CAD build for the part. Positions are in the model's coordinates, mm. A direction names the side the tool comes from. Round coordinates to 2 decimals unless told otherwise and drop trailing zeros. Write each loop counter-clockwise with the first axis right and the second up, starting at its lowest first coordinate (ties: lowest second). Pieces come first, ordered by that corner, then holes. Notation, with made-up numbers: (12, 15.25) - (37, 15.25) arc R19 ccw to (37, 47.25) - close; hole circle Ø6 at (45.25, -29.75). An arc over 180 degrees is marked (long way). Use one line per item in the form item = value. Start each with the question number.
Item 1: Drill centre line: L1, parallel to Z at x = -90, y = 5.75. Where is it in solid material? Low to high.
Item 2: Band-saw the part on A-A, the plane x = -224.5. List the corners of the cut face in (y, z).
Item 3: Pull direction X, two halves, no side cores. Call faces 1 (the flat face through (-108.74, 3, 73)), 2 (the flat face through (-357, 3, -69.85)), 3 (the flat face through (-360.818, 3, 1)): +X half, -X half, draft (parallel to the pull), parting line (faces both ways), or undercut.
Item 4: Pin check, flat tips, straight feed: pin 1 (1.9 mm diameter, centred on y = 4.5, z = 74, fed in from -X); pin 2 (1.9 mm diameter, centred on y = 2, z = 72.5, fed in from +X); pin 3 (3 mm diameter, centred on x = -356.5, y = 3.5, fed in from -Z). Stop position of each tip, or through.
Item 5: Tool access for faces 4 (the flat face through (-288.119, 3, 73)), 5 (the flat face through (-353.198, 3, -73)), 6 (the flat face through (-33, 3, 76.2)), 7 (the flat face through (-308, 3, -69.85)), 8 (the flat face through (-187, 3, -76.2)): list every direction of +Z, -Z, +X, -X, +Y, -Y with a clear straight run to the whole face (end or side of a thin tool).
from build123d import *

# Parameters (mm, degrees)
SKETCH1_W                 = 721.63658441
SKETCH1_H                 = 152.4
BOSS_EXTRUDE1_DEPTH       = 6.35
SKETCH2_W                 = 39.679316882
SKETCH2_H                 = 6.35
SKETCH2_W_2               = 31.750000127
CUT_EXTRUDE1_DEPTH        = 7.35
LPATTERN1_COUNT           = 3
LPATTERN1_PITCH           = 153.979316882
LPATTERN1_COL_COUNT       = 3
LPATTERN1_COL_PITCH       = 153.979316882
MIRROR1_COPY_1_SKETCH_W   = 39.679316882
MIRROR1_COPY_1_SKETCH_H   = 6.35
MIRROR1_COPY_1_SKETCH_W_2 = 31.750000127
MIRROR1_COPY_1_DEPTH      = 7.35
MIRROR1_COPY_2_SKETCH_W   = 39.679316882
MIRROR1_COPY_2_SKETCH_H   = 6.35
MIRROR1_COPY_2_SKETCH_W_2 = 31.750000127
MIRROR1_COPY_2_DEPTH      = 7.35
MIRROR1_COPY_3_SKETCH_W   = 39.679316882
MIRROR1_COPY_3_SKETCH_H   = 6.35
MIRROR1_COPY_3_SKETCH_W_2 = 31.750000127
MIRROR1_COPY_3_DEPTH      = 7.35
MIRROR1_COPY_4_SKETCH_W   = 39.679316882
MIRROR1_COPY_4_SKETCH_H   = 6.35
MIRROR1_COPY_4_SKETCH_W_2 = 31.750000127
MIRROR1_COPY_4_DEPTH      = 7.35
SKETCH4_W                 = 360.818292205
SKETCH4_H                 = 152.4
CUT_EXTRUDE2_DEPTH        = 7.35


with BuildPart() as part:
    # Sketch1 → Boss-Extrude1 (new body)
    with BuildSketch(Plane(origin=(0, 0, 0), x_dir=(1, 0, 0), z_dir=(0, 1, 0))):
        Rectangle(SKETCH1_W, SKETCH1_H)
    extrude(amount=BOSS_EXTRUDE1_DEPTH)

    # Sketch2 → Cut-Extrude1 (cut, through all)
    with BuildSketch(Plane(origin=(0, 6.35, 0), x_dir=(1, 0, 0), z_dir=(0, 1, 0))):
        with Locations((0, -73.025)):
            Rectangle(SKETCH2_W, SKETCH2_H)
        with Locations((-61.114658505, -73.025)):
            Rectangle(SKETCH2_W_2, SKETCH2_H)
        with Locations((61.114658505, -73.025)):
            Rectangle(SKETCH2_W_2, SKETCH2_H)
    cut_extrude1 = extrude(amount=-CUT_EXTRUDE1_DEPTH, mode=Mode.SUBTRACT)

    # LPattern1: Cut-Extrude1 ×3
    with Locations(*[(i * LPATTERN1_PITCH, 0, 0) for i in range(1, LPATTERN1_COUNT)]):
        add(cut_extrude1, mode=Mode.SUBTRACT)

    # LPattern1 col: Cut-Extrude1 ×3
    with Locations(*[(-i * LPATTERN1_COL_PITCH, 0, 0) for i in range(1, LPATTERN1_COL_COUNT)]):
        add(cut_extrude1, mode=Mode.SUBTRACT)

    # Mirror1: Cut-Extrude1 across plane
    add(cut_extrude1.mirror(Plane.XY), mode=Mode.SUBTRACT)

    # Mirror1 copy 1 sketch → Mirror1 copy 1 (cut, through all)
    with BuildSketch(Plane(origin=(153.979316882, 6.35, 0), x_dir=(1, 0, 0), z_dir=(0, 1, 0))):
        with Locations((0, 73.025)):
            Rectangle(MIRROR1_COPY_1_SKETCH_W, MIRROR1_COPY_1_SKETCH_H)
        with Locations((-61.114658505, 73.025)):
            Rectangle(MIRROR1_COPY_1_SKETCH_W_2, MIRROR1_COPY_1_SKETCH_H)
        with Locations((61.114658505, 73.025)):
            Rectangle(MIRROR1_COPY_1_SKETCH_W_2, MIRROR1_COPY_1_SKETCH_H)
    extrude(amount=-MIRROR1_COPY_1_DEPTH, mode=Mode.SUBTRACT)

    # Mirror1 copy 2 sketch → Mirror1 copy 2 (cut, through all)
    with BuildSketch(Plane(origin=(307.958633764, 6.35, 0), x_dir=(1, 0, 0), z_dir=(0, 1, 0))):
        with Locations((0, 73.025)):
            Rectangle(MIRROR1_COPY_2_SKETCH_W, MIRROR1_COPY_2_SKETCH_H)
        with Locations((-61.114658505, 73.025)):
            Rectangle(MIRROR1_COPY_2_SKETCH_W_2, MIRROR1_COPY_2_SKETCH_H)
        with Locations((61.114658505, 73.025)):
            Rectangle(MIRROR1_COPY_2_SKETCH_W_2, MIRROR1_COPY_2_SKETCH_H)
    extrude(amount=-MIRROR1_COPY_2_DEPTH, mode=Mode.SUBTRACT)

    # Mirror1 copy 3 sketch → Mirror1 copy 3 (cut, through all)
    with BuildSketch(Plane(origin=(-153.979316882, 6.35, 0), x_dir=(1, 0, 0), z_dir=(0, 1, 0))):
        with Locations((0, 73.025)):
            Rectangle(MIRROR1_COPY_3_SKETCH_W, MIRROR1_COPY_3_SKETCH_H)
        with Locations((-61.114658505, 73.025)):
            Rectangle(MIRROR1_COPY_3_SKETCH_W_2, MIRROR1_COPY_3_SKETCH_H)
        with Locations((61.114658505, 73.025)):
            Rectangle(MIRROR1_COPY_3_SKETCH_W_2, MIRROR1_COPY_3_SKETCH_H)
    extrude(amount=-MIRROR1_COPY_3_DEPTH, mode=Mode.SUBTRACT)

    # Mirror1 copy 4 sketch → Mirror1 copy 4 (cut, through all)
    with BuildSketch(Plane(origin=(-307.958633764, 6.35, 0), x_dir=(1, 0, 0), z_dir=(0, 1, 0))):
        with Locations((0, 73.025)):
            Rectangle(MIRROR1_COPY_4_SKETCH_W, MIRROR1_COPY_4_SKETCH_H)
        with Locations((-61.114658505, 73.025)):
            Rectangle(MIRROR1_COPY_4_SKETCH_W_2, MIRROR1_COPY_4_SKETCH_H)
        with Locations((61.114658505, 73.025)):
            Rectangle(MIRROR1_COPY_4_SKETCH_W_2, MIRROR1_COPY_4_SKETCH_H)
    extrude(amount=-MIRROR1_COPY_4_DEPTH, mode=Mode.SUBTRACT)

    # Sketch4 → Cut-Extrude2 (cut, through all)
    with BuildSketch(Plane(origin=(0, 6.35, 0), x_dir=(1, 0, 0), z_dir=(0, 1, 0))):
        with Locations((180.409146103, 0)):
            Rectangle(SKETCH4_W, SKETCH4_H)
    extrude(amount=-CUT_EXTRUDE2_DEPTH, mode=Mode.SUBTRACT)


solid = part.part
Determined:
q1.L1 = -69.85 to 69.85
q2.outline = (0, -69.85) - (6.35, -69.85) - (6.35, 69.85) - (0, 69.85) - close
q3.face_1 = undercut
q3.face_2 = draft
q3.face_3 = -X half
q4.pin_1 = -353.2
q4.pin_2 = -19.84
q4.pin_3 = -69.85
q5.face_4 = +Z, +Y, -Y
q5.face_5 = -Z, -X, +Y, -Y
q5.face_6 = +Z, +X, -X, +Y, -Y
q5.face_7 = -Z, +Y, -Y
q5.face_8 = -Z, +X, -X, +Y, -Y
